Here's the drawing with two shaded views (mm, measured from the low corner). I have some questions. Round coordinates to 2 decimals unless told otherwise and drop trailing zeros. Loops run counter-clockwise (first coordinate to the right, second up) from the corner with the lowest first, then second, coordinate; pieces in that order, holes last. Notation, with made-up numbers: (33.5, -15) -> (77.5, -15) arc R27 ccw to (77.5, 20) -> close; hole circle Ø4 at (33.25, 14). An arc over 180 degrees is marked (long way). Use a Markdown table: item, result.
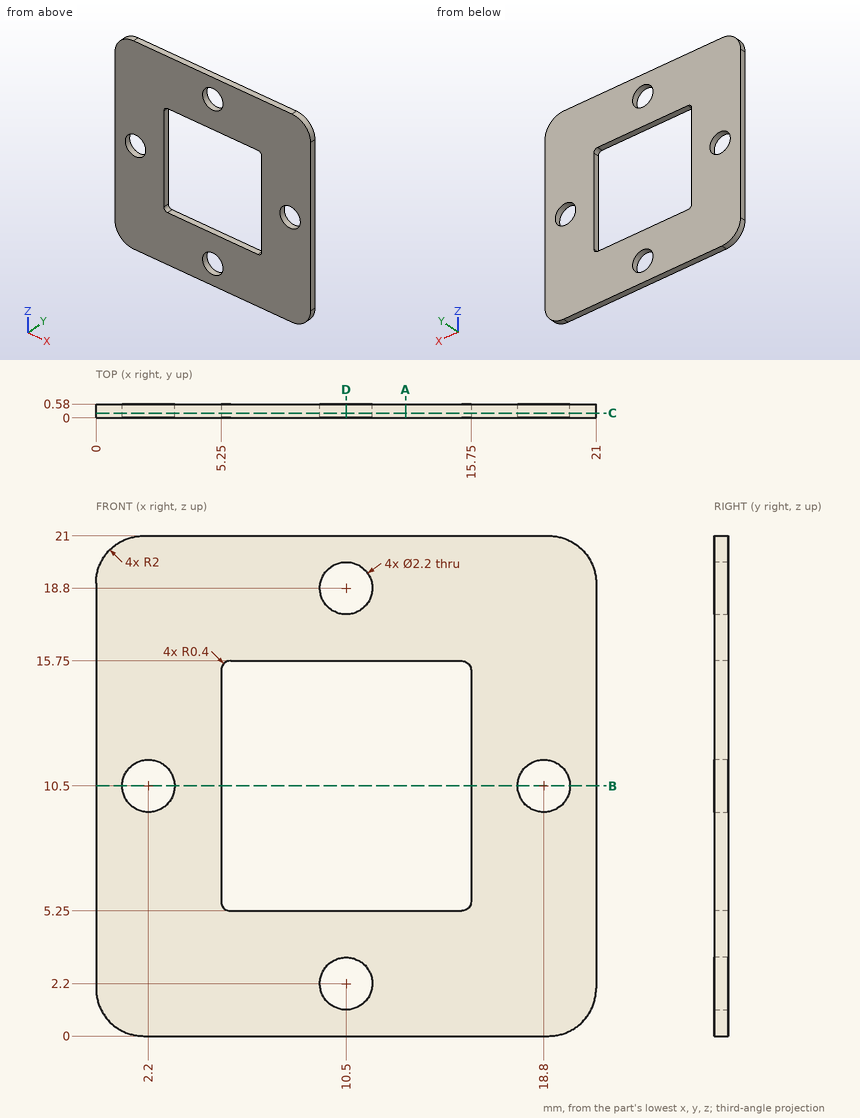
1. Will this pin go through, and if not, where does the flat tip stop? pin 1 Ø12 at (x, z) = (8.5, 2.5) entering from -Y.
Answer sheet:
| item | result |
|---|---|
| pin 1 | stops at y = 0 |
2. I want a section at A-A (x = 13). Please give me the cut outline in (y, z), plus the area to 3 significant figures.
Answer sheet:
| item | result |
|---|---|
| outline | (0, 0) -> (0.58, 0) -> (0.58, 5.25) -> (0, 5.25) -> close; (0, 15.75) -> (0.58, 15.75) -> (0.58, 21) -> (0, 21) -> close |
| area | 6.09 mm² |
3. I want a section at B-B (z = 10.5). Please give me the cut outline in (x, y).
Answer sheet:
| item | result |
|---|---|
| outline | (0, 0) -> (1.1, 0) -> (1.1, 0.58) -> (0, 0.58) -> close; (3.3, 0) -> (5.25, 0) -> (5.25, 0.58) -> (3.3, 0.58) -> close; (15.75, 0) -> (17.7, 0) -> (17.7, 0.58) -> (15.75, 0.58) -> close; (19.9, 0) -> (21, 0) -> (21, 0.58) -> (19.9, 0.58) -> close |
4. I need wall thicknesses on line 1 (X direction, y = 0.3, z = 10.5); line 2 (X direction, y = 0.2, z = 18.8); line 3 (Z direction, x = 14.5, y = 0.1). Which ranges of each line are inside material? Lowest first, please.
Answer sheet:
| item | result |
|---|---|
| line 1 | x = 0 to 1.1, 3.3 to 5.25, 15.75 to 17.7, 19.9 to 21 |
| line 2 | x = 0 to 9.4, 11.6 to 21 |
| line 3 | z = 0 to 5.25, 15.75 to 21 |
5. I want a section at D-D (x = 10.5). Please give me the cut outline in (y, z).
Answer sheet:
| item | result |
|---|---|
| outline | (0, 0) -> (0.58, 0) -> (0.58, 1.1) -> (0, 1.1) -> close; (0, 3.3) -> (0.58, 3.3) -> (0.58, 5.25) -> (0, 5.25) -> close; (0, 15.75) -> (0.58, 15.75) -> (0.58, 17.7) -> (0, 17.7) -> close; (0, 19.9) -> (0.58, 19.9) -> (0.58, 21) -> (0, 21) -> close |
6. I want a section at C-C (y = 0.2). Please give me the cut outline in (x, z).
Answer sheet:
| item | result |
|---|---|
| outline | (0, 2) arc R2 ccw to (2, 0) -> (19, 0) arc R2 ccw to (21, 2) -> (21, 19) arc R2 ccw to (19, 21) -> (2, 21) arc R2 ccw to (0, 19) -> close; hole circle Ø2.2 at (2.2, 10.5); hole (5.25, 5.65) arc R0.4 ccw to (5.65, 5.25) -> (15.35, 5.25) arc R0.4 ccw to (15.75, 5.65) -> (15.75, 15.35) arc R0.4 ccw to (15.35, 15.75) -> (5.65, 15.75) arc R0.4 ccw to (5.25, 15.35) -> close; hole circle Ø2.2 at (10.5, 2.2); hole circle Ø2.2 at (10.5, 18.8); hole circle Ø2.2 at (18.8, 10.5) |
